Geometry: final body of the model. Coordinates: model frame, mm. A direction names the side the tool comes from. Coordinates: 2 decimals unless noted, no trailing zeros. Order: outer loops, then holes, each group sorted by start corner. A loop starts at its lowest first (then second) coordinate and runs counter-clockwise, first axis right, second up. Notation, with made-up numbers: M 59,30 L 99,30 A22 ccw 99,38 Z; hole C 26,-38.75 d2. An arc over 180 degrees is marked long. Use CSV: the item, a comma, the result in double quotes. Start each with the question number.
Q1. Section query C-C, the plane x = 0. Output: boundary loops of the cut face in (y, z), and give its area (3 significant figures).
Q2. Ray query, probe 1 along Y at (x, z) = (-10, 0.8); probe 2 along Z at (x, y) = (-8, 5); probe 3 along Z at (x, y) = (13, 1.5). Return the intervals inside material, ascending.
Q3. Access query for faces 1 (the face through (-4.95, 2.91, 8.13)), 2 (the face through (-5, 0, 0)). Directions: +Z, -Z, +X, -X, +Y, -Y. A direction counts if a zero-diameter tool reaches every point of the face in a straight line with its end or side. Return the directions, or none.
Q4. First-contact query: P1, Ø5, axis at x = 0, y = 0, coming from the -Z side; P2, Ø2, axis at x = 1.5, z = 6.5, coming from the +Y side; P3, Ø7, axis at x = 10, y = 0, coming from the -Z side; P4, Ø3.5, axis at x = -1.5, z = 8, coming from the -Y side. Flat tips, straight axial feed; report the tip coordinate or a pass-through.
Q5. Section query A-A, the plane x = 10. Output: boundary loops of the cut face in (y, z), and give its area (3 significant figures).
Q6. Section query B-B, the plane z = 12. Output: boundary loops of the cut face in (x, y), and give its area (3 significant figures).
Q7. Mould query, pull axis Y, two halves, no side actions, for faces 3 (the face through (13, 0, 1.5)), 4 (the face through (19.55, 9.57, 1.62)), 5 (the face through (-7, 0, 1.5)), 6 (the face through (0, -10, 2)). Classes: +Y half, -Y half, draft (parallel to the pull), parting line (faces both ways), or undercut.
Q8. Section query D-D, the plane y = -7.75. Output: boundary loops of the cut face in (x, z).
from build123d import *

# Parameters (mm, degrees)
SKETCH_W        = 40
SKETCH_H        = 20
SKETCH_R        = 2.75
PAD_DEPTH       = 3.2
FILLET_R        = 1.5
PAD001_DEPTH    = 10
SKETCH002_R     = 4
POCKET_DEPTH    = 13.201
SKETCH003_R     = 4.5
POCKET001_DEPTH = 1.5
CHAMFER_SIZE    = 0.3
CHAMFER001_SIZE = 0.3


with BuildPart() as part:
    # Sketch → Pad (new body)
    with BuildSketch(Plane.XY):
        Rectangle(SKETCH_W, SKETCH_H)
        with Locations((10, 0)):
            Circle(SKETCH_R, mode=Mode.SUBTRACT)
        with Locations((-10, 0)):
            Circle(SKETCH_R, mode=Mode.SUBTRACT)
    extrude(amount=PAD_DEPTH)

    # Fillet
    fillet_edges = [part.edges().sort_by_distance(p)[0] for p in [
        (-20, -10, 1.6),
        (-20, 10, 1.6),
        (20, 10, 1.6),
        (20, -10, 1.6),
    ]]
    fillet(fillet_edges, radius=FILLET_R)

    # Sketch001 (on Face5 of Fillet) → Pad001 (join)
    with BuildSketch(Plane.XY.offset(3.2)):
        Polygon((6.627981, 0), (3.313991, 5.74), (-3.313991, 5.74), (-6.627981, 0), (-3.313991, -5.74), (3.313991, -5.74), align=None)
    extrude(amount=PAD001_DEPTH)

    # Sketch002 (on Face19 of Pad001) → Pocket (cut, through all)
    with BuildSketch(Plane.XY.offset(13.2)):
        Circle(SKETCH002_R)
    extrude(amount=-POCKET_DEPTH, mode=Mode.SUBTRACT)

    # Sketch003 (on Face2 of Pocket) → Pocket001 (cut)
    with BuildSketch(Plane(origin=(0, 0, 0), x_dir=(1, 0, 0), z_dir=(0, 0, -1))):
        with Locations((10, 0)):
            Circle(SKETCH003_R)
        with Locations((-10, 0)):
            Circle(SKETCH003_R)
    extrude(amount=-POCKET001_DEPTH, mode=Mode.SUBTRACT)

    # Chamfer
    chamfer_edges = [part.edges().sort_by_distance(p)[0] for p in [
        (5.5, 0, 0),
        (-4, 0, 0),
        (-14.5, 0, 0),
    ]]
    chamfer(chamfer_edges, length=CHAMFER_SIZE)

    # Chamfer001
    chamfer001_edges = [part.edges().sort_by_distance(p)[0] for p in [
        (4.970986, 2.87, 3.2),
        (-4, 0, 13.2),
        (-12.75, 0, 3.2),
    ]]
    chamfer(chamfer001_edges, length=CHAMFER001_SIZE)


solid = part.part
Responses:
1,outline,"M -10,0 L -4.3,0 L -4,0.3 L -4,12.9 L -4.3,13.2 L -5.74,13.2 L -5.74,3.2 L -10,3.2 Z; M 4,0.3 L 4.3,0 L 10,0 L 10,3.2 L 5.74,3.2 L 5.74,13.2 L 4.3,13.2 L 4,12.9 Z"
1,area,"73.0 mm²"
2,probe 1,"y = -10 to -4.5, 4.5 to 10"
2,probe 2,"z = 0 to 3.2"
2,probe 3,"z = 1.5 to 3.2"
3,face 1,"+Z, -X, +Y"
3,face 2,"-Z, +X, -X, +Y, -Y"
4,P1,"passes through"
4,P2,"stops at y = 5.74"
4,P3,"stops at z = 1.5"
4,P4,"stops at y = -5.74"
5,outline,"M -10,0 L -4.8,0 L -4.5,0.3 L -4.5,1.5 L -2.75,1.5 L -2.75,3.2 L -10,3.2 Z; M 2.75,1.5 L 4.5,1.5 L 4.5,0.3 L 4.8,0 L 10,0 L 10,3.2 L 2.75,3.2 Z"
5,area,"41.1 mm²"
6,outline,"M -6.63,0 L -3.31,-5.74 L 3.31,-5.74 L 6.63,0 L 3.31,5.74 L -3.31,5.74 Z; hole C 0,0 d8"
6,area,"63.9 mm²"
7,face 3,"undercut"
7,face 4,"+Y half"
7,face 5,"undercut"
7,face 6,"-Y half"
8,outline,"M -20,0 L 20,0 L 20,3.2 L -20,3.2 Z"
